Work out the finished part from the listing and answer in its coordinate system (mm). A direction names the side the tool comes from. Round coordinates to 2 decimals unless told otherwise and drop trailing zeros. Order: outer loops, then holes, each group sorted by start corner. A loop starts at its lowest first (then second) coordinate and runs counter-clockwise, first axis right, second up. Notation, with made-up numbers: (43.25, -36.5) -> (83.25, -36.5) arc R24 ccw to (83.25, -0.5) -> close; hole circle Ø9 at (85, 55). An arc over 180 degrees is marked (long way). Use one line per item in the form item = value.
```python
from build123d import *

# Parameters (mm, degrees)
SKETCH_1_W          = 52
SKETCH_1_H          = 28
EXTRUDE_1_DEPTH     = 5
SKETCH_2_R          = 17.5
EXTRUDE_2_DEPTH     = 5
SKETCH_3_R          = 15
EXTRUDE_3_DEPTH     = 8
SKETCH_4_R          = 13
CUT_EXTRUDE_1_DEPTH = 34.930075155
FILLET_1_R          = 10
SKETCH_5_R          = 2
CUT_EXTRUDE_2_DEPTH = 34.930075155
FILLET_2_R          = 1
FILLET_3_R          = 1
FILLET_4_R          = 1


with BuildPart() as part:
    # 草圖1 → 填料-伸長1 (new body)
    with BuildSketch(Plane(origin=(0, 0, 0), x_dir=(1, 0, 0), z_dir=(0, 1, 0))):
        Rectangle(SKETCH_1_W, SKETCH_1_H)
    extrude(amount=EXTRUDE_1_DEPTH)

    # 草圖2 → 填料-伸長2 (add)
    with BuildSketch(Plane(origin=(0, 0, 0), x_dir=(1, 0, 0), z_dir=(0, 1, 0))):
        Circle(SKETCH_2_R)
    extrude(amount=EXTRUDE_2_DEPTH)

    # 草圖3 → 填料-伸長3 (add)
    with BuildSketch(Plane(origin=(0, 5, 0), x_dir=(1, 0, 0), z_dir=(0, 1, 0))):
        with Locations(Location((0, 0, 0), (0, 0, 270))):
            Circle(SKETCH_3_R)
    extrude(amount=EXTRUDE_3_DEPTH)

    # 草圖4 → 除料-伸長1 (cut, through all)
    with BuildSketch(Plane(origin=(0, 13, 0), x_dir=(1, 0, 0), z_dir=(0, 1, 0))):
        with Locations(Location((0, 0, 0), (0, 0, 270))):
            Circle(SKETCH_4_R)
    extrude(amount=-CUT_EXTRUDE_1_DEPTH, mode=Mode.SUBTRACT)

    # 圓角1
    fillet_1_edges = [part.edges().sort_by_distance(p)[0] for p in [
        (-26, 2.5, -14),
        (26, 2.5, -14),
        (26, 2.5, 14),
        (-26, 2.5, 14),
    ]]
    fillet(fillet_1_edges, radius=FILLET_1_R)

    # 草圖5 → 除料-伸長2 (cut, through all)
    with BuildSketch(Plane.XZ):
        with Locations(Location((-21, 0, 0), (0, 0, 270))):
            Circle(SKETCH_5_R)
    cut_extrude_2 = extrude(amount=-CUT_EXTRUDE_2_DEPTH, mode=Mode.SUBTRACT)

    # 鏡射1: 除料-伸長2 across plane
    add(cut_extrude_2.mirror(Plane(origin=(0, 0, 0), x_dir=(0, 0, 1), z_dir=(1, 0, 0))), mode=Mode.SUBTRACT)

    # 圓角2
    fillet_2_edges = [part.edges().sort_by_distance(p)[0] for p in [
        (0, 5, -15),
    ]]
    fillet(fillet_2_edges, radius=FILLET_2_R)

    # 圓角3
    fillet_3_edges = [part.edges().sort_by_distance(p)[0] for p in [
        (10.5, 2.5, 14),
        (-10.5, 2.5, 14),
        (-10.5, 2.5, -14),
        (10.5, 2.5, -14),
    ]]
    fillet(fillet_3_edges, radius=FILLET_3_R)

    # 圓角4
    fillet_4_edges = [part.edges().sort_by_distance(p)[0] for p in [
        (13.414101957, 5, -14),
        (26, 5, 0),
        (-26, 5, 0),
        (-13.414101957, 5, 14),
        (-23.071067812, 5, -11.071067812),
        (-23.071067812, 5, 11.071067812),
        (23.071067812, 5, 11.071067812),
        (23.071067812, 5, -11.071067812),
        (0, 5, -17.5),
        (-13.414101957, 5, -14),
        (0, 5, 17.5),
        (13.414101957, 5, 14),
        (10.520641571, 5, -14.048472068),
        (-10.520641571, 5, -14.048472068),
        (-10.520641571, 5, 14.048472068),
        (10.520641571, 5, 14.048472068),
    ]]
    fillet(fillet_4_edges, radius=FILLET_4_R)


solid = part.part
```
Item 1: The part is cut by section C-C, the plane z = 0. Give the vertices of the cut face in (x, y), and give its area (3 significant figures).
Findings:
outline = (-26, 0) -> (-23, 0) -> (-23, 5) -> (-25, 5) arc R1 ccw to (-26, 4) -> close; (-19, 0) -> (-13, 0) -> (-13, 13) -> (-15, 13) -> (-15, 6) arc R1 cw to (-16, 5) -> (-19, 5) -> close; (13, 0) -> (19, 0) -> (19, 5) -> (16, 5) arc R1 cw to (15, 6) -> (15, 13) -> (13, 13) -> close; (23, 0) -> (26, 0) -> (26, 4) arc R1 ccw to (25, 5) -> (23, 5) -> close
area = 122 mm^2
Item 2: Consider line 1 along X through (y, z) = (1.9, 0); line 2 along X through (y, z) = (5.5, 0); line 3 along X through (y, z) = (6.5, 3). Determine where each line is inside the solid, lowest interval first.
Findings:
line_1 = -26 to -23, -19 to -13, 13 to 19, 23 to 26
line_2 = -15.13 to -13, 13 to 15.13
line_3 = -14.7 to -12.65, 12.65 to 14.7
Item 3: For faces 1 (the cylindrical face through (13.45, 4.715, -13.699)), 2 (the cylindrical face through (-13.378, 4.715, -13.699)), 3 (the flat face through (13, 2, 14)), determine the directions among +Z, -Z, +X, -X, +Y, -Y from which every point of the face is accessible in a straight line to the end or side of a thin tool.
Findings:
face_1 = -Z, +X, +Y
face_2 = -Z, -X, +Y
face_3 = +Z, +X, +Y, -Y
Item 4: Determine the mould class of faces 4 (the flat face through (13, 2, -14)), 5 (the cylindrical face through (19, 2, 0)), 6 (the cylindrical face through (-19, 2, 0)), 7 (the flat face through (-13, 2, 14)) for opening direction Z: released by +Z, released by -Z, zero draft, split by the parting line, or undercut.
Findings:
face_4 = released by -Z
face_5 = undercut
face_6 = undercut
face_7 = released by +Z
Item 5: The part is cut by section B-B, the plane y = 2.25. Give the vertices of the cut face in (x, z), and give its area (3 significant figures).
Findings:
outline = (-26, -4) arc R10 ccw to (-16, -14) -> (-10.83, -14) arc R1 cw to (-10.24, -14.19) arc R17.5 ccw to (10.24, -14.19) arc R1 cw to (10.83, -14) -> (16, -14) arc R10 ccw to (26, -4) -> (26, 4) arc R10 ccw to (16, 14) -> (10.83, 14) arc R1 cw to (10.24, 14.19) arc R17.5 ccw to (-10.24, 14.19) arc R1 cw to (-10.83, 14) -> (-16, 14) arc R10 ccw to (-26, 4) -> close; hole circle Ø4 at (-21, 0); hole circle Ø26 at (0, 0); hole circle Ø4 at (21, 0)
area = 914 mm^2
Item 6: The part is cut by section A-A, the plane x = 0. Give the vertices of the cut face in (y, z), and give its area (3 significant figures).
Findings:
outline = (0, -17.5) -> (4, -17.5) arc R1 ccw to (5, -16.5) -> (5, -16) arc R1 cw to (6, -15) -> (13, -15) -> (13, -13) -> (0, -13) -> close; (0, 13) -> (13, 13) -> (13, 15) -> (6, 15) arc R1 cw to (5, 16) -> (5, 16.5) arc R1 ccw to (4, 17.5) -> (0, 17.5) -> close
area = 77.0 mm^2
Item 7: Flat-ended cylindrical pins translate along their axes: P1, Ø1.5, axis at y = 11.5, z = 13, coming from the +X side; P2, Ø5, axis at y = 5, z = 12.5, coming from the +X side; P3, Ø4.5, axis at x = -14.5, y = 3, coming from the -Z side. Find the tip coordinate at first contact, or state that the pin passes through.
Findings:
P1 = 8.66
P2 = 23.87
P3 = -14
Item 8: The part is cut by section D-D, the plane y = 10. Give the vertices of the cut face in (x, z).
Findings:
outline = circle Ø30 at (0, 0); hole circle Ø26 at (0, 0)
